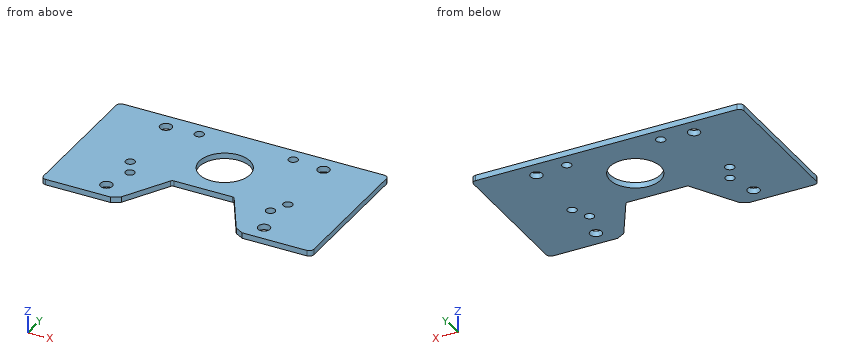
from build123d import *

# Parameters (mm, degrees)
SKETCH1_R           = 2.6035
SKETCH1_R_2         = 3.3655
SKETCH1_R_3         = 14.2875
BOSS_EXTRUDE1_DEPTH = 3.175
SKETCH2_W           = 25.4
SKETCH2_H           = 82.55
BOSS_EXTRUDE2_DEPTH = 3.175
FILLET1_R           = 2.54


with BuildPart() as part:
    # Sketch1 → Boss-Extrude1 (new body)
    with BuildSketch(Plane.XY.offset(3.175)):
        with BuildLine():
            Line((53.975, -25.4), (53.975, 50.8))
            Line((53.975, 50.8), (50.8, 53.975))
            Line((50.8, 53.975), (-50.8, 53.975))
            Line((-50.8, 53.975), (-53.975, 50.8))
            Line((-53.975, 50.8), (-53.975, -25.4))
            Line((-53.975, -25.4), (-50.8, -28.575))
            Line((-50.8, -28.575), (-37.135283942, -28.575))
            Line((-37.135283942, -28.575), (-32.372783942, -25.825369343))
            Line((-32.372783942, -25.825369343), (-17.920771776, -0.79375))
            ThreePointArc((-17.920771776, -0.79375), (-17.339706448, -0.212684671), (-16.545956448, 0))
            Line((-16.545956448, 0), (16.545956448, 0))
            ThreePointArc((16.545956448, 0), (17.339706448, -0.212684671), (17.920771776, -0.79375))
            Line((17.920771776, -0.79375), (32.372783942, -25.825369343))
            Line((32.372783942, -25.825369343), (37.135283942, -28.575))
            Line((37.135283942, -28.575), (50.8, -28.575))
            Line((50.8, -28.575), (53.975, -25.4))
        make_face()
        with Locations((44.45, 6.35)):
            Circle(SKETCH1_R, mode=Mode.SUBTRACT)
        with Locations((26.484101205, 46.005749811)):
            Circle(SKETCH1_R, mode=Mode.SUBTRACT)
        with Locations((-39.632108696, -3.063282164)):
            Circle(SKETCH1_R, mode=Mode.SUBTRACT)
        with Locations((44.45, -19.05)):
            Circle(SKETCH1_R_2, mode=Mode.SUBTRACT)
        with Locations((44.45, 44.45)):
            Circle(SKETCH1_R_2, mode=Mode.SUBTRACT)
        with Locations((0, 23.058733918)):
            Circle(SKETCH1_R_3, mode=Mode.SUBTRACT)
        with Locations((-44.45, 44.45)):
            Circle(SKETCH1_R_2, mode=Mode.SUBTRACT)
        with Locations((-44.45, -19.05)):
            Circle(SKETCH1_R_2, mode=Mode.SUBTRACT)
        with Locations((-44.45, 6.35)):
            Circle(SKETCH1_R, mode=Mode.SUBTRACT)
        with Locations((-26.484101205, 46.005749811)):
            Circle(SKETCH1_R, mode=Mode.SUBTRACT)
        with Locations((39.632108696, -3.063282164)):
            Circle(SKETCH1_R, mode=Mode.SUBTRACT)
    extrude(amount=-BOSS_EXTRUDE1_DEPTH)

    # Sketch2 → Boss-Extrude2 (add, through all)
    with BuildSketch(Plane.XY.offset(3.175)):
        with Locations((-63.5, 12.7)):
            Rectangle(SKETCH2_W, SKETCH2_H)
        with Locations((63.5, 12.7)):
            Rectangle(SKETCH2_W, SKETCH2_H)
    extrude(amount=-BOSS_EXTRUDE2_DEPTH)

    # Fillet1
    fillet1_edges = [part.edges().sort_by_distance(p)[0] for p in [
        (76.2, -28.575, 1.5875),
        (76.2, 53.975, 1.5875),
        (-76.2, -28.575, 1.5875),
        (-76.2, 53.975, 1.5875),
    ]]
    fillet(fillet1_edges, radius=FILLET1_R)


solid = part.part
Geometry check sheet. Reference: the model listing, model coordinates, mm. Coordinates: 2 decimals unless noted, no trailing zeros. Loops run counter-clockwise (first coordinate to the right, second up) from the corner with the lowest first, then second, coordinate; pieces in that order, holes last. Notation, with made-up numbers: (-17.75, 14.5) - (31.25, 14.5) arc R31 ccw to (31.25, 46.5) - close; hole circle Ø1 at (85.5, 21). An arc over 180 degrees is marked (long way). Use one line per item in the form item = value. Start each with the question number.
Item 1: Section check A-A, the plane y = 6.35. Enter the section's corners in (x, z) (1 decimal).
Item 2: Gauge pin test, flat ends, axial feed: pin 1 (11 mm diameter, centred on x = -44.45, y = -19.05, fed in from -Z); pin 2 (1.5 mm diameter, centred on x = -26, z = 2, fed in from -Y); pin 3 (1.6 mm diameter, centred on x = 4, z = 1, fed in from -Y). Record the tip position at first contact, or that the pin passes through.
Item 3: Section check D-D, the plane y = -19.05. Enter the section's corners in (x, z) (1 decimal), and give its area (3 significant figures).
Item 4: Section check C-C, the plane x = 44.45. Enter the section's corners in (y, z) (1 decimal).
Item 5: Thickness scan on probe 1 along Y at (x, z) = (-44.45, 1.55) (1 decimal); probe 2 along X at (y, z) = (8.5, 0.85); probe 3 along X at (y, z) = (44, 1.65). Record the ranges inside material, lowest first.
Item 6: Section check B-B, the plane x = 0. Enter the section's corners in (y, z) (3 decimals), and give its area (3 significant figures).
Computed:
q1.outline = (-76.2, 0) - (-47.1, 0) - (-47.1, 3.2) - (-76.2, 3.2) - close; (-41.8, 0) - (41.8, 0) - (41.8, 3.2) - (-41.8, 3.2) - close; (47.1, 0) - (76.2, 0) - (76.2, 3.2) - (47.1, 3.2) - close
q2.pin_1 = 0
q2.pin_2 = -16.09
q2.pin_3 = 0
q3.outline = (-76.2, 0) - (-47.8, 0) - (-47.8, 3.2) - (-76.2, 3.2) - close; (-41.1, 0) - (-28.5, 0) - (-28.5, 3.2) - (-41.1, 3.2) - close; (28.5, 0) - (41.1, 0) - (41.1, 3.2) - (28.5, 3.2) - close; (47.8, 0) - (76.2, 0) - (76.2, 3.2) - (47.8, 3.2) - close
q3.area = 260 mm2
q4.outline = (-28.6, 0) - (-22.4, 0) - (-22.4, 3.2) - (-28.6, 3.2) - close; (-15.7, 0) - (3.7, 0) - (3.7, 3.2) - (-15.7, 3.2) - close; (9, 0) - (41.1, 0) - (41.1, 3.2) - (9, 3.2) - close; (47.8, 0) - (54, 0) - (54, 3.2) - (47.8, 3.2) - close
q5.probe_1 = -28.6 to -22.4, -15.7 to 3.7, 9 to 41.1, 47.8 to 54
q5.probe_2 = -76.2 to -45.92, -42.98 to 42.98, 45.92 to 76.2
q5.probe_3 = -76.2 to -47.79, -41.11 to -28.14, -24.82 to 24.82, 28.14 to 41.11, 47.79 to 76.2
q6.outline = (0, 0) - (8.771, 0) - (8.771, 3.175) - (0, 3.175) - close; (37.346, 0) - (53.975, 0) - (53.975, 3.175) - (37.346, 3.175) - close
q6.area = 80.6 mm2
